Could you check a few things on this model? Use its own coordinates, in mm. Give positions to 0.01 mm unless a question says otherwise; leave off trailing zeros. Order: outer loops, then holes, each group sorted by start corner. A loop starts at its lowest first (then second) coordinate and runs counter-clockwise, first axis right, second up. Notation, with made-up numbers: M 23,-24.5 L 54,-24.5 A23 ccw 54,-11.5 Z; hole C 49.5,18.5 d4. An arc over 180 degrees is marked long. Return JSON: item names as keys, results as strings. Group by question number.
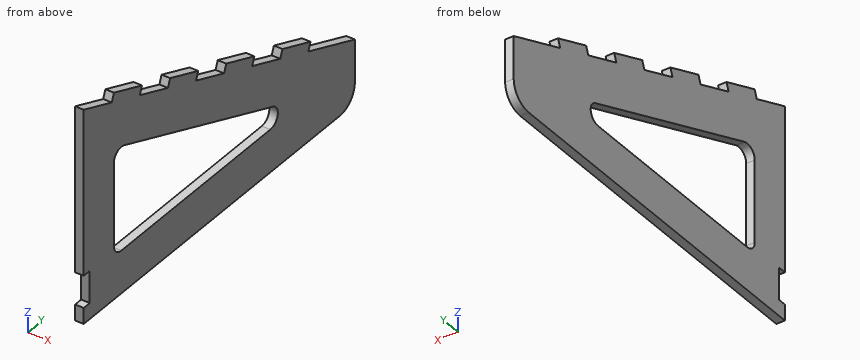
```python
from build123d import *

# Parameters (mm, degrees)
ESTRUSIONE_ESTRUSIONE1_DEPTH = 4
ESTRUSIONE_ESTRUSIONE2_DEPTH = 4
RACCORDO2_R                  = 10
RACCORDO3_R                  = 5


with BuildPart() as part:
    # Schizzo1 → Estrusione-Estrusione1 (new body)
    with BuildSketch(Plane(origin=(0, 0, 0), x_dir=(0, 0, -1), z_dir=(1, 0, 0))):
        Polygon((70, 180), (0, 0), (77.5, 0), (77.5, 4), (92.5, 4), (92.5, 0), (100, 0), (100, 180), align=None)
        Polygon((80, 150.533691669), (80, 20), (29.236897684, 20), align=None, mode=Mode.SUBTRACT)
    extrude(amount=ESTRUSIONE_ESTRUSIONE1_DEPTH)

    # Schizzo2 → Estrusione-Estrusione2 (add)
    with BuildSketch(Plane(origin=(4, 0, 0), x_dir=(0, 0, -1), z_dir=(1, 0, 0))):
        Polygon((7.248925223, 18.640093431), (3.520906537, 20.089878475), (10.76983176, 38.729971906), (14.497850446, 37.280186862), align=None)
        Polygon((28.995700892, 74.560373723), (21.746775669, 55.920280292), (18.018756983, 57.370065337), (25.267682206, 76.010158768), align=None)
        Polygon((43.493551339, 111.840560585), (36.244626115, 93.200467154), (32.516607429, 94.650252199), (39.765532652, 113.29034563), align=None)
        Polygon((57.991401785, 149.120747447), (50.742476562, 130.480654016), (47.014457876, 131.93043906), (54.263383099, 150.570532491), align=None)
    extrude(amount=-ESTRUSIONE_ESTRUSIONE2_DEPTH)

    # Raccordo2
    raccordo2_edges = [part.edges().sort_by_distance(p)[0] for p in [
        (2, 180, -100),
    ]]
    fillet(raccordo2_edges, radius=RACCORDO2_R)

    # Raccordo3
    raccordo3_edges = [part.edges().sort_by_distance(p)[0] for p in [
        (2, 20, -80),
        (2, 150.533691669, -80),
        (2, 20, -29.236897684),
    ]]
    fillet(raccordo3_edges, radius=RACCORDO3_R)


solid = part.part
```
1. Imagine slicing it at D-D, the plane z = -87.5. Please give me the cut outline in (x, y).
2. Imagine slicing it at A-A, the plane z = -61.5. Please give me the cut outline in (x, y).
3. For pin 1 (2 mm diameter, centred on x = 1, z = -85, fed in from -Y); pin 2 (2 mm diameter, centred on x = 2, y = 2, fed in from +Z), each with a flat end and sliding along its axis, tell me the tip position at first contact or that it passes through.
4. Imagine slicing it at C-C, the plane y = 85. Please give me the cut outline in (x, z).
5. I need wall thicknesses on L1, parallel to Y at x = 2.55, z = -74.5; L2, parallel to Z at x = 3.8, y = 54; L3, parallel to Z at x = 0.8, y = 114. Which ranges of each line are inside material? Lowest first, please. Write a range as from..to.
Values:
{
 "1": {"outline": "M 0,4 L 4,4 L 4,180 L 0,180 Z"},
 "2": {"outline": "M 0,0 L 4,0 L 4,20 L 0,20 Z; M 0,102.96 L 4,102.96 L 4,158.14 L 0,158.14 Z"},
 "3": {"pin 1": "stops at y = 4", "pin 2": "stops at z = -0.39"},
 "4": {"outline": "M 0,-100 L 4,-100 L 4,-80 L 0,-80 Z; M 0,-54.51 L 4,-54.51 L 4,-33.06 L 0,-33.06 Z"},
 "5": {"L1": "y = 0..20, 128.86..180", "L2": "z = -100..-80, -42.46..-21", "L3": "z = -100..-80, -65.79..-44.33"}
}
